Autodesk Fusion 360 part; units mm, degrees
sketch "スケッチ1" plane through (0, 0, 0) normal (0, 1, 0) x (1, 0, 0)
  circle A0 centre (0, 0) radius 14
  circle A1 centre (0, 0) radius 9.5 construction
  line L0 (-9.5, 0) -> (9.5, 0) construction
  circle A2 centre (-9.5, 0) radius 1.175
  circle A3 centre (9.5, 0) radius 1.175
  circle A4 centre (0, 0) radius 12.5 construction
  line L1 (0, 12.5) -> (0, -12.5) construction
  circle A5 centre (0, 12.5) radius 1.175
  circle A6 centre (0, -12.5) radius 1.175
  dimension "d1" = 28
  dimension "d2" = 19
  dimension "d3" = 2.35
  dimension "d4" = 2.35
  dimension "d5" = 25
  dimension "d6" = 2.35
  dimension "d7" = 2.35
extrude "押し出し1" add sketch "スケッチ1" along normal blind 2 contours A2 | A3 | A5 | A6 makes body 1 at (1.1735, 1.3333, -12.4414) makes body 2 at (-8.3265, 1.3333, 0.0586) makes body 3 at (10.6735, 1.3333, 0.0586) makes body 4 at (1.1735, 1.3333, 12.5586)
extrude "押し出し2" add sketch "スケッチ1" against normal blind 4 contours A0 | A2 | A3 | A5 | A6 bodies 1 2 3 4
sketch "スケッチ2" plane through (0, -4, 0) normal (0, -1, 0) x (1, 0, 0)
  circle A0 centre (0, 0) radius 14
  circle A1 centre (0, 0) radius 4
  dimension "d12" = 8
extrude "押し出し3" cut sketch "スケッチ2" against normal blind 4 contours A1 bodies 1
ref_plane "作業平面1" through (0, -2, 0) normal (0, -1, 0) x (-1, 0, 0)
sketch "スケッチ3" plane through (0, -2, 0) normal (0, -1, 0) x (-1, 0, 0)
  circle A0 centre (0, 0) radius 4
  circle A1 centre (0, 0) radius 3.45
  dimension "d16" = 8
  dimension "d17" = 6.9
extrude "押し出し4" add sketch "スケッチ3" along normal blind 3 bodies 1
ref_plane "作業平面3" through (0, -4, 0) normal (0, -1, 0) x (-1, 0, 0)
sketch "スケッチ5" plane through (0, -4, 0) normal (0, -1, 0) x (-1, 0, 0)
  circle A0 centre (0, 0) radius 3.45
  circle A1 centre (0, 0) radius 3.15
  dimension "d26" = 6.9
  dimension "d27" = 6.3
extrude "押し出し6" add sketch "スケッチ5" along normal blind 1 bodies 1
extrude "押し出し7" add 1 faces at (10.6145, -4, 0.6955) along direction (0, -1, 0) blind 1 on bodies 1 bodies 1
Verification items for the finished model (mm, model axes). A direction names the side the tool comes from. Give positions to 0.01 mm unless a question says otherwise; leave off trailing zeros. Loops run counter-clockwise (first coordinate to the right, second up) from the corner with the lowest first, then second, coordinate; pieces in that order, holes last.
1) Sectioned sample at A-A, the plane x = 0. Enter the section's corners in (y, z) (3 decimals).
2) Sectioned sample at B-B, the plane z = 0. Enter the section's corners in (x, y) (3 decimals), then the cut area to 3 significant figures.
3) Sectioned sample at C-C, the plane y = 0.75. Enter the section's corners in (x, z) (3 decimals), then the cut area to 3 significant figures.
4) Set-up check for faces 4 (the cylindrical face through (0.45, -2.99, 3.42)), 5 (the flat face through (-10, 2, 0)): record each of +Z, -Z, +X, -X, +Y, -Y from which the full face is reachable in a straight line by a thin tool's end or side.
5) Thickness scan on line 1 along X through (y, z) = (-0.55, 0); line 2 along Z through (x, y) = (0, -4.6). Record the ranges inside material, lowest first.
6) Sectioned sample at D-D, the plane z = 12.5. Enter the section's corners in (x, y) (3 decimals), then the cut area to 3 significant figures.
7) Draft check along Z on faces 1 (the flat face through (0, 2, -13)), 2 (the cylindrical face through (-10.674, 0.986, 0.052)), 3 (the cylindrical face through (-0.867, -1.014, -3.905)). Enter one of: pulls with the +Z half, pulls with the -Z half, needs draft (parallel to the pull), parting line crosses it, or undercut.
8) Depth check by flat-ended pin: pin 1 Ø8 at (x, z) = (9, -6) entering from +Y; pin 2 Ø5 at (x, z) = (0, 0) entering from +Y; pin 3 Ø6.5 at (x, z) = (0, 0) entering from +Y. Enter the tip coordinate at first touch or a pass-through.
Answers:
1. outline: (-5, -14) - (0, -14) - (0, -13.675) - (2, -13.675) - (2, -11.325) - (0, -11.325) - (0, -4) - (-2, -4) - (-2, -3.45) - (-4, -3.45) - (-4, -3.15) - (-5, -3.15) - close; (-5, 3.15) - (-4, 3.15) - (-4, 3.45) - (-2, 3.45) - (-2, 4) - (0, 4) - (0, 11.325) - (2, 11.325) - (2, 13.675) - (0, 13.675) - (0, 14) - (-5, 14) - close
2. outline: (-14, -5) - (-3.15, -5) - (-3.15, -4) - (-3.45, -4) - (-3.45, -2) - (-4, -2) - (-4, 0) - (-8.325, 0) - (-8.325, 2) - (-10.675, 2) - (-10.675, 0) - (-14, 0) - close; (3.15, -5) - (14, -5) - (14, 0) - (10.675, 0) - (10.675, 2) - (8.325, 2) - (8.325, 0) - (4, 0) - (4, -2) - (3.45, -2) - (3.45, -4) - (3.15, -4) - close
2. area: 113 mm2
3. outline: circle Ø2.35 at (-9.5, 0); circle Ø2.35 at (0, -12.5); circle Ø2.35 at (0, 12.5); circle Ø2.35 at (9.5, 0)
3. area: 17.3 mm2
4. face 4: +Y
4. face 5: +Z, -Z, +X, -X, +Y
5. line 1: x = -14 to -4, 4 to 14
5. line 2: z = -14 to -3.15, 3.15 to 14
6. outline: (-6.305, -5) - (6.305, -5) - (6.305, 0) - (1.175, 0) - (1.175, 2) - (-1.175, 2) - (-1.175, 0) - (-6.305, 0) - close
6. area: 67.7 mm2
7. face 1: needs draft
7. face 2: parting line crosses it
7. face 3: undercut
8. pin 1: stops at y = 0
8. pin 2: passes through
8. pin 3: stops at y = -4
